```python
from build123d import *

# Parameters (mm, degrees)
F1_DEPTH = 12.7


with BuildPart() as f1:
    # F0 (on Front) → F1 (new body)
    with BuildSketch(Plane.XZ):
        with BuildLine():
            Line((150.283333, 25.311652), (-1.058333, 12.655826))
            ThreePointArc((-1.058333, 12.655826), (-12.7, 0), (-1.058333, -12.655826))
            Line((-1.058333, -12.655826), (150.283333, -25.311652))
            ThreePointArc((150.283333, -25.311652), (177.8, 0), (150.283333, 25.311652))
        make_face()
        with BuildLine():
            ThreePointArc((-0.79375, -9.491869), (-9.525, 0), (-0.79375, 9.491869))
            Line((-0.79375, 9.491869), (150.547917, 22.147695))
            ThreePointArc((150.547917, 22.147695), (167.446396, 16.357157), (174.625, 0))
            ThreePointArc((174.625, 0), (167.446396, -16.357157), (150.547917, -22.147695))
            Line((150.547917, -22.147695), (-0.79375, -9.491869))
        make_face(mode=Mode.SUBTRACT)
    extrude(amount=F1_DEPTH)


solid = f1.part
```
The model under review builds one solid part; all positions refer to its coordinate system, in mm. A direction names the side the tool comes from. Give positions to 0.01 mm unless a question says otherwise; leave off trailing zeros. Write each loop counter-clockwise with the first axis right and the second up, starting at its lowest first coordinate (ties: lowest second). Pieces come first, ordered by that corner, then holes.
(1) To check wall thickness, follow L1, parallel to X at y = -1.5, z = -1; L2, parallel to X at y = -2.25, z = 7; L3, parallel to Z at x = 88, y = -1.5. State the ranges of each line that lie inside material, in increasing order.
(2) Consider section A-A, the plane x = 152.4. Give the boundary of the cut face in (y, z) (3 decimals), and give its area (3 significant figures).
(3) For P1, Ø1, axis at x = 79.5, y = -2, coming from the +Z side; P2, Ø3, axis at x = 121, y = -10, coming from the +Z side; P3, Ø2, axis at y = -4.5, z = -9, coming from the +X side; P4, Ø4, axis at x = 70.5, z = 17.5, coming from the +Y side, all flat-tipped, find the tip position at first contact; note any pin that passes through.
(4) The part is to be moulded in two halves that separate along Z. For faces 1 (the flat face through (82, -12.7, -17)), 2 (the flat face through (73.82, -6.26, 15.73)), 3 (the cylindrical face through (-12.697, -6.261, 0.264)), say which applies: released by +Z, released by -Z, zero draft, split by the parting line, or undercut.
(5) Consider section C-C, the plane z = 20. Give the boundary of the cut face in (x, y).
(6) Consider section B-B, the plane y = -8. Give the boundary of the cut face in (x, z) (3 decimals), and give its area (3 significant figures).
(7) Tool access review of faces 4 (the flat face through (75.94, -6.26, -15.91)), 5 (the flat face through (82, 0, -17)): name each direction out of +Z, -Z, +X, -X, +Y, -Y from which nothing blocks a thin tool from reaching the whole face with its end or side.
Returned:
1. L1: x = -12.66 to -9.47, 174.6 to 177.78
1. L2: x = -10.6 to -6.46, 173.49 to 176.82
1. L3: z = -20.1 to -16.92, 16.92 to 20.1
2. outline: (-12.7, -25.4) - (0, -25.4) - (0, -22.225) - (-12.7, -22.225) - close; (-12.7, 22.225) - (0, 22.225) - (0, 25.4) - (-12.7, 25.4) - close
2. area: 80.6 mm2
3. P1: stops at z = 19.43
3. P2: stops at z = 22.99
3. P3: stops at x = 176.51
3. P4: stops at y = 0
4. face 1: zero draft
4. face 2: undercut
4. face 3: split by the parting line
5. outline: (86.77, -12.7) - (124.87, -12.7) - (124.87, 0) - (86.77, 0) - close; (162.09, -12.7) - (168.06, -12.7) - (168.06, 0) - (162.09, 0) - close
6. outline: (-1.058, -12.656) - (150.283, -25.312) arc R25.4 ccw (long way) to (150.283, 25.312) - (-1.058, 12.656) arc R12.7 ccw to start; hole (-0.794, -9.492) - (150.548, -22.148) arc R22.225 ccw (long way) to (150.548, 22.148) - (-0.794, 9.492) arc R9.525 ccw to start
6. area: 1,320 mm2
7. face 4: +Y, -Y
7. face 5: +Z, -Z, +X, -X, +Y
